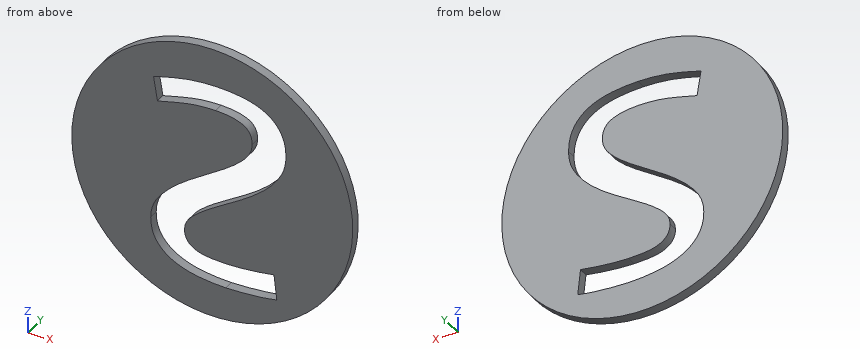
from build123d import *

# Parameters (mm, degrees)
SKETCH1_R           = 45
BOSS_EXTRUDE1_DEPTH = 3


with BuildPart() as part:
    # Sketch1 → Boss-Extrude1 (new body)
    with BuildSketch(Plane(origin=(0, 0, 0), x_dir=(1, 0, 0), z_dir=(0, 1, 0))):
        with Locations(Location((0, 0, 0), (0, 0, 270))):  # turned: the seam where the file's is
            Circle(SKETCH1_R)
        with BuildLine():
            add(Edge.make_bspline(
                [(19.780990946, 24.185124764), (19.255065107, 24.287914798), (18.122086305, 24.509350826), (16.316551627, 24.770179957), (14.357752418, 25.057330128), (12.311058297, 25.302832973), (10.229567608, 25.537930243), (8.173301101, 25.696077882), (6.221913509, 25.819266557), (4.969956895, 25.839869106), (4.377345112, 25.849621292)],
                knots=[0, 0, 0, 0, 0.829036243, 1.785956155, 2.822045536, 3.89228551, 4.975307857, 6.062841547, 7.083048955, 8, 8, 8, 8], degree=3))
            add(Edge.make_bspline(
                [(4.377345112, 25.849621292), (3.446204146, 25.839565028), (1.65716034, 25.820243466), (-0.523497459, 25.678422406), (-2.134814502, 25.466621363), (-3.234258723, 25.269743374), (-4.239722547, 24.96405185), (-5.163089497, 24.614993657), (-6.002431575, 24.201660489), (-6.733506828, 23.675895663), (-7.383141898, 23.092997796), (-7.930081052, 22.419543279), (-8.359935091, 21.657367799), (-8.673790899, 20.796588784), (-8.856015855, 19.829357364), (-8.873240581, 19.150114951), (-8.882203499, 18.796669903)],
                knots=[0, 0, 0, 0, 2.295489194, 4.410428573, 5.380894891, 6.301560079, 7.159764947, 7.966985716, 8.734184816, 9.457764993, 10.179765198, 10.880326743, 11.586237622, 12.32697511, 13.129438398, 14, 14, 14, 14], degree=3))
            add(Edge.make_bspline(
                [(-8.882203499, 18.796669903), (-8.850818027, 18.360202528), (-8.787076829, 17.473774773), (-8.299529285, 16.177773231), (-7.531705877, 14.918174723), (-6.468835972, 13.707430879), (-5.199588079, 12.505820488), (-3.750460779, 11.316874284), (-2.173501164, 10.095772106), (0.19047217, 8.465461016), (3.392591141, 6.389097084), (7.401158074, 3.84423487), (11.436980484, 1.154437496), (14.598547163, -1.337138932), (16.941188197, -3.441782617), (18.524295541, -5.116615111), (19.962389169, -6.861115679), (21.249269366, -8.677300905), (22.30079899, -10.59536019), (23.087128729, -12.62347507), (23.521482235, -14.771077168), (23.585470219, -16.235887567), (23.617796501, -16.975899541)],
                knots=[0, 0, 0, 0, 0.519213468, 1.054477964, 1.630134935, 2.270161266, 2.967727746, 3.71175636, 4.503051278, 5.34407491, 7.13300234, 9.051150551, 11.003302341, 12.910294161, 13.842483047, 14.754150315, 15.653890787, 16.535313878, 17.40293064, 18.254252337, 19.118060482, 20, 20, 20, 20], degree=3))
            add(Edge.make_bspline(
                [(23.617796501, -16.975899541), (23.599786365, -17.672825423), (23.564928796, -19.021684862), (23.270802134, -20.965503255), (22.762650283, -22.748577872), (22.050483541, -24.36572214), (21.174041496, -25.835244154), (20.110888209, -27.14506), (18.897414426, -28.327096204), (17.50009469, -29.336609406), (15.962883146, -30.226180167), (14.258614821, -30.943249705), (12.420117395, -31.575353637), (10.428945987, -32.043245685), (8.315670511, -32.386430983), (6.098422851, -32.63922249), (3.77777338, -32.797342644), (2.195888092, -32.819567974), (1.386893723, -32.830934264)],
                knots=[0, 0, 0, 0, 1.075194104, 2.080975546, 3.024934148, 3.928271024, 4.800677613, 5.657461563, 6.524782954, 7.407242198, 8.310928775, 9.259978089, 10.255920614, 11.308444205, 12.411965724, 13.558733007, 14.751507922, 16, 16, 16, 16], degree=3))
            add(Edge.make_bspline(
                [(1.386893723, -32.830934264), (0.384854835, -32.819567929), (-1.579565413, -32.797285102), (-4.469689043, -32.557780783), (-7.246791058, -32.207577643), (-9.885005378, -31.670272649), (-12.368606742, -31.076733402), (-14.681000089, -30.469055859), (-16.813387105, -29.868409154), (-18.164915503, -29.439515535), (-18.812759054, -29.233929055)],
                knots=[0, 0, 0, 0, 1.166641361, 2.287110747, 3.375174177, 4.42434953, 5.420457035, 6.34882319, 7.208522552, 8, 8, 8, 8], degree=3))
            Line((-18.812759054, -29.233929055), (-17.557333707, -21.391047111))
            add(Edge.make_bspline(
                [(-17.557333707, -21.391047111), (-16.92765023, -21.571066227), (-15.623509008, -21.943904896), (-13.597987784, -22.494044975), (-11.428021788, -23.040422446), (-9.137280734, -23.613361679), (-6.72469763, -24.121615317), (-4.205720245, -24.443757714), (-1.60294269, -24.668864111), (0.163871673, -24.693436806), (1.062457959, -24.705934264)],
                knots=[0, 0, 0, 0, 0.82784923, 1.714563499, 2.653014331, 3.656340952, 4.699592855, 5.767128945, 6.864381369, 8, 8, 8, 8], degree=3))
            add(Edge.make_bspline(
                [(1.062457959, -24.705934264), (1.876650637, -24.687246807), (3.435097114, -24.651477141), (5.663708681, -24.375253087), (7.66548934, -23.896733066), (9.185584763, -23.345151534), (10.24171498, -22.753709402), (10.937316717, -22.248785046), (11.499265321, -21.629257743), (11.979043163, -20.941428467), (12.342776891, -20.163357249), (12.596885499, -19.297650342), (12.751136892, -18.354355508), (12.773133718, -17.695897336), (12.784463168, -17.356758916)],
                knots=[0, 0, 0, 0, 1.865164993, 3.57011294, 5.132569067, 6.57499646, 7.255114939, 7.901464084, 8.534112646, 9.161604161, 9.81695743, 10.491765748, 11.223185006, 12, 12, 12, 12], degree=3))
            add(Edge.make_bspline(
                [(12.784463168, -17.356758916), (12.752373418, -16.859917427), (12.687880197, -15.861377146), (12.224204459, -14.388468451), (11.462465357, -12.964292087), (10.390925154, -11.60553121), (9.124414869, -10.267841999), (7.686118718, -8.936597872), (6.095227969, -7.612559939), (3.717571546, -5.85406476), (0.52885577, -3.635742908), (-3.489713573, -1.025376634), (-7.505368863, 1.697395276), (-10.696639338, 4.119771578), (-13.043162038, 6.168454152), (-14.637770832, 7.740654265), (-16.064077212, 9.372166101), (-17.348452609, 11.025867113), (-18.42180964, 12.766347784), (-19.168862671, 14.625642809), (-19.624536603, 16.58376369), (-19.684854205, 17.919645128), (-19.715536832, 18.599187264)],
                knots=[0, 0, 0, 0, 0.591380666, 1.188542884, 1.822507787, 2.505918877, 3.243027329, 4.015898054, 4.839248524, 5.707487546, 7.538026587, 9.466039613, 11.415971731, 13.317280673, 14.234172866, 15.125381555, 15.982728632, 16.814024653, 17.618094752, 18.409678073, 19.191027939, 20, 20, 20, 20], degree=3))
            add(Edge.make_bspline(
                [(-19.715536832, 18.599187264), (-19.69007572, 19.296431103), (-19.640869758, 20.643919536), (-19.294531368, 22.582084159), (-18.679144546, 24.338232741), (-17.842869563, 25.923663704), (-16.779110741, 27.326321286), (-15.558622534, 28.586881396), (-14.182283058, 29.714351392), (-12.623789919, 30.673268851), (-10.917968821, 31.496846545), (-9.069476595, 32.208414475), (-7.081002803, 32.779480609), (-4.958515074, 33.227140213), (-2.733752509, 33.556420942), (-0.422428367, 33.79150112), (1.95338712, 33.958539874), (3.563608319, 33.969222666), (4.377345112, 33.974621292)],
                knots=[0, 0, 0, 0, 1.03838471, 2.006774832, 2.919286264, 3.799627568, 4.665221273, 5.531947435, 6.40804449, 7.307755042, 8.250508454, 9.225938019, 10.254284747, 11.328399385, 12.454517948, 13.602227205, 14.788268378, 16, 16, 16, 16], degree=3))
            add(Edge.make_bspline(
                [(4.377345112, 33.974621292), (5.110989126, 33.965254351), (6.607281613, 33.946150149), (8.869481458, 33.827722709), (11.14014177, 33.657276118), (13.354931043, 33.460072759), (15.4510663, 33.250532473), (17.378136504, 32.963398675), (19.099276185, 32.65905252), (20.171790498, 32.430381936), (20.669662821, 32.324230667)],
                knots=[0, 0, 0, 0, 1.073469456, 2.189378298, 3.313843796, 4.405133658, 5.442979297, 6.395522168, 7.255184668, 8, 8, 8, 8], degree=3))
            Line((20.669662821, 32.324230667), (19.780990946, 24.185124764))
        make_face(mode=Mode.SUBTRACT)
    extrude(amount=BOSS_EXTRUDE1_DEPTH)


solid = part.part
Model file for the job. Use its own axes, mm. Round coordinates to 2 decimals unless told otherwise and drop trailing zeros. Order: outer loops, then holes, each group sorted by start corner. A loop starts at its lowest first (then second) coordinate and runs counter-clockwise, first axis right, second up.
(1) Band-saw the part on B-B (x = -21). List the corners of the cut face in (y, z), then the cut area to 3 significant figures.
(2) Band-saw the part on A-A (x = 0). Give the number of separate pieces and of enclosed holes in the cut face, then the cut area to 3 significant figures.
(3) Drill centre lines: line 1 (Z direction, x = -2.5, y = 2.3); line 2 (Z direction, x = 11.5, y = 2); line 3 (X direction, y = 2.9, z = -18). Where is each one in solid material? Low to high.
Verdict:
1. outline: (0, -39.8) - (3, -39.8) - (3, 39.8) - (0, 39.8) - close
1. area: 239 mm2
2. separate pieces: 4
2. enclosed holes: 0
2. area: 186 mm2
3. line 1: z = -44.93 to -33.57, -25.4 to -10.36, 1.66 to 24.58, 32.71 to 44.93
3. line 2: z = -43.51 to -33.62, -25.39 to -1.03, 13.11 to 21.6, 31.78 to 43.51
3. line 3: x = -41.24 to -19.69, -8.81 to 41.24
